```python
from build123d import *

# Parameters (mm, degrees)
SKETCH1_R           = 2.5
BOSS_EXTRUDE1_DEPTH = 1.5
BOSS_EXTRUDE2_DEPTH = 3.5


with BuildPart() as part:
    # Sketch1 → Boss-Extrude1 (new body)
    with BuildSketch(Plane.XY):
        with BuildLine():
            Line((39.75, 20), (-39.75, 20))
            ThreePointArc((-39.75, 20), (-40.457106781, 19.707106781), (-40.75, 19))
            Line((-40.75, 19), (-40.75, -19))
            ThreePointArc((-40.75, -19), (-40.457106781, -19.707106781), (-39.75, -20))
            Line((-39.75, -20), (39.75, -20))
            ThreePointArc((39.75, -20), (40.457106781, -19.707106781), (40.75, -19))
            Line((40.75, -19), (40.75, 19))
            ThreePointArc((40.75, 19), (40.457106781, 19.707106781), (39.75, 20))
        make_face()
        with Locations((-36.375, 16)):
            Circle(SKETCH1_R, mode=Mode.SUBTRACT)
        with Locations((-4.375, 16)):
            Circle(SKETCH1_R, mode=Mode.SUBTRACT)
        with Locations((-4.375, -16)):
            Circle(SKETCH1_R, mode=Mode.SUBTRACT)
        with Locations((-36.375, -16)):
            Circle(SKETCH1_R, mode=Mode.SUBTRACT)
        with Locations(Location((36.375, -16, 0), (0, 0, 180))):
            Circle(SKETCH1_R, mode=Mode.SUBTRACT)
        with Locations(Location((4.375, -16, 0), (0, 0, 180))):
            Circle(SKETCH1_R, mode=Mode.SUBTRACT)
        with Locations(Location((4.375, 16, 0), (0, 0, 180))):
            Circle(SKETCH1_R, mode=Mode.SUBTRACT)
        with Locations(Location((36.375, 16, 0), (0, 0, 180))):
            Circle(SKETCH1_R, mode=Mode.SUBTRACT)
        with BuildLine():
            Line((26.619997998, 19), (14.130002002, 19))
            ThreePointArc((14.130002002, 19), (5.767776688, 13.661223485), (1, 4.960783708))
            Line((1, 4.960783708), (1, -4.960783708))
            ThreePointArc((1, -4.960783708), (5.767776688, -13.661223485), (14.130002002, -19))
            Line((14.130002002, -19), (26.619997998, -19))
            ThreePointArc((26.619997998, -19), (34.982223312, -13.661223485), (39.75, -4.960783708))
            Line((39.75, -4.960783708), (39.75, 4.960783708))
            ThreePointArc((39.75, 4.960783708), (34.982223312, 13.661223485), (26.619997998, 19))
        make_face(mode=Mode.SUBTRACT)
        with BuildLine():
            Line((-39.75, 4.960783708), (-39.75, -4.960783708))
            ThreePointArc((-39.75, -4.960783708), (-34.982223312, -13.661223485), (-26.619997998, -19))
            Line((-26.619997998, -19), (-14.130002002, -19))
            ThreePointArc((-14.130002002, -19), (-5.767776688, -13.661223485), (-1, -4.960783708))
            Line((-1, -4.960783708), (-1, 4.960783708))
            ThreePointArc((-1, 4.960783708), (-5.767776688, 13.661223485), (-14.130002002, 19))
            Line((-14.130002002, 19), (-26.619997998, 19))
            ThreePointArc((-26.619997998, 19), (-34.982223312, 13.661223485), (-39.75, 4.960783708))
        make_face(mode=Mode.SUBTRACT)
    extrude(amount=BOSS_EXTRUDE1_DEPTH)

    # Sketch2 → Boss-Extrude2 (add)
    with BuildSketch(Plane(origin=(0, 0, 0), x_dir=(-1, 0, 0), z_dir=(0, 0, -1))):
        with BuildLine():
            Line((39.75, 22), (-39.75, 22))
            ThreePointArc((-39.75, 22), (-41.871320344, 21.121320344), (-42.75, 19))
            Line((-42.75, 19), (-42.75, -19))
            ThreePointArc((-42.75, -19), (-41.871320344, -21.121320344), (-39.75, -22))
            Line((-39.75, -22), (39.75, -22))
            ThreePointArc((39.75, -22), (41.871320344, -21.121320344), (42.75, -19))
            Line((42.75, -19), (42.75, 19))
            ThreePointArc((42.75, 19), (41.871320344, 21.121320344), (39.75, 22))
        make_face()
        with BuildLine():
            Line((40.75, -19), (40.75, 19))
            ThreePointArc((40.75, 19), (40.457106781, 19.707106781), (39.75, 20))
            Line((39.75, 20), (-39.75, 20))
            ThreePointArc((-39.75, 20), (-40.457106781, 19.707106781), (-40.75, 19))
            Line((-40.75, 19), (-40.75, -19))
            ThreePointArc((-40.75, -19), (-40.457106781, -19.707106781), (-39.75, -20))
            Line((-39.75, -20), (39.75, -20))
            ThreePointArc((39.75, -20), (40.457106781, -19.707106781), (40.75, -19))
        make_face(mode=Mode.SUBTRACT)
    extrude(amount=-BOSS_EXTRUDE2_DEPTH)


solid = part.part
```
The listing builds one solid part. Answer for the finished solid, in the listing's coordinates (mm). A direction names the side the tool comes from. Coordinates: 2 decimals unless noted, no trailing zeros. Loops run counter-clockwise (first coordinate to the right, second up) from the corner with the lowest first, then second, coordinate; pieces in that order, holes last. Notation, with made-up numbers: (68.5, 61.25) -> (91.5, 61.25) arc R29 ccw to (91.5, 88.25) -> close; hole circle Ø6 at (52.25, 17.5). An arc over 180 degrees is marked (long way). Return JSON: item names as keys, results as strings. Group by question number.
(1) A cutting plane is placed at C-C on y = 16. Count the separate pieces of the cut face and the enclosed holes in it, and give its area (4 significant figures).
(2) Determine the mould class of faces 1 (the cylindrical face through (41.85, 21.14, 1.73)), 2 (the flat face through (20, 19, 1)), 3 (the cylindrical face through (-41.85, -21.14, 1.73)) for opening direction X: released by +X, released by -X, zero draft, split by the parting line, or undercut.
(3) Which of the six approach directions +Z, -Z, +X, -X, +Y, -Y give full straight-line access (tool end or side, diameter ignored) to faces 4 (the flat face through (3, -21, 3.5)), 5 (the cylindrical face through (5.9, 13.8, 0.7))?
(4) A cutting plane is placed at A-A on x = 35. Write down the section's boundary in (y, z).
(5) Given pin 1 Ø4 at (x, y) = (4.375, -16) entering from -Z; pin 2 Ø6.5 at (x, y) = (36.375, 16) entering from +Z, each flat-ended and moving along its own axis, determine where each tip first touches the part or whether it passes through.
(6) A cutting plane is placed at B-B on y = 1. Write down the section's boundary in (x, z).
(7) A cutting plane is placed at D-D on x = -10.5. Write down the section's boundary in (y, z).
(8) Find the intervals of material crossed by probe 1 along Y at (x, z) = (-17, 1.1); probe 2 along Y at (x, z) = (36, 2.8); probe 3 along X at (y, z) = (3, 3.35), in increasing order. Write a range as from..to.
The answers:
{
 "1": {"separate pieces": "7", "enclosed holes": "0", "area": "34.25 mm^2"},
 "2": {"face 1": "released by +X", "face 2": "undercut", "face 3": "released by -X"},
 "3": {"face 4": "+Z, +X, -X, +Y, -Y", "face 5": "+Z, -Z"},
 "4": {"outline": "(-22, 0) -> (-18.09, 0) -> (-18.09, 1.5) -> (-20, 1.5) -> (-20, 3.5) -> (-22, 3.5) -> close; (-13.91, 0) -> (-13.64, 0) -> (-13.64, 1.5) -> (-13.91, 1.5) -> close; (13.64, 0) -> (13.91, 0) -> (13.91, 1.5) -> (13.64, 1.5) -> close; (18.09, 0) -> (22, 0) -> (22, 3.5) -> (20, 3.5) -> (20, 1.5) -> (18.09, 1.5) -> close"},
 "5": {"pin 1": "passes through", "pin 2": "stops at z = 1.5"},
 "6": {"outline": "(-42.75, 0) -> (-39.75, 0) -> (-39.75, 1.5) -> (-40.75, 1.5) -> (-40.75, 3.5) -> (-42.75, 3.5) -> close; (-1, 0) -> (1, 0) -> (1, 1.5) -> (-1, 1.5) -> close; (39.75, 0) -> (42.75, 0) -> (42.75, 3.5) -> (40.75, 3.5) -> (40.75, 1.5) -> (39.75, 1.5) -> close"},
 "7": {"outline": "(-22, 0) -> (-17.39, 0) -> (-17.39, 1.5) -> (-20, 1.5) -> (-20, 3.5) -> (-22, 3.5) -> close; (17.39, 0) -> (22, 0) -> (22, 3.5) -> (20, 3.5) -> (20, 1.5) -> (17.39, 1.5) -> close"},
 "8": {"probe 1": "y = -22..-19, 19..22", "probe 2": "y = -22..-20, 20..22", "probe 3": "x = -42.75..-40.75, 40.75..42.75"}
}
